Part model, mm, in its own coordinate system. Face numbers are marked on the shaded views. A direction names the side the tool comes from. Give positions to 0.01 mm unless a question says otherwise; leave off trailing zeros. Loops run counter-clockwise (first coordinate to the right, second up) from the corner with the lowest first, then second, coordinate; pieces in that order, holes last. Notation, with made-up numbers: M -7,22.5 L 50,22.5 A19 ccw 50,33.5 Z; hole C 35.25,3.25 d3. An arc over 180 degrees is marked long. Answer in a Markdown table with one row per item.
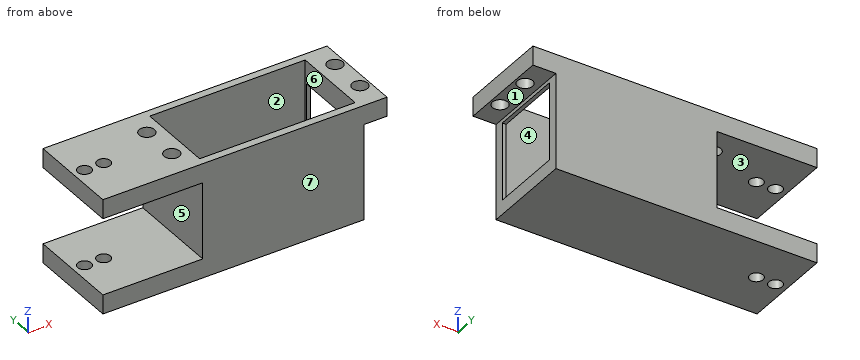
from build123d import *

# Parameters (mm, degrees)
SKETCH1_W                 = 56
SKETCH1_H                 = 24
BOSS_EXTRUDE1_DEPTH       = 30
SHELL1_T                  = -2
SHELL1_THICKNESS_2_FACE_W = 28
SHELL1_THICKNESS_2_FACE_H = 20
SHELL1_THICKNESS_2_DEPTH  = 6.5
SHELL1_THICKNESS_3_FACE_W = 28
SHELL1_THICKNESS_3_FACE_H = 20
SHELL1_THICKNESS_3_DEPTH  = 5
SKETCH12_W                = 20
SKETCH12_H                = 19
CUT_EXTRUDE1_DEPTH        = 10
FILLET1_R                 = 2
SKETCH13_W                = 2
SKETCH13_H                = 24
CUT_EXTRUDE2_DEPTH        = 43.755116653
SKETCH17_W                = 25
SKETCH17_H                = 24
CUT_EXTRUDE4_DEPTH        = 4
SKETCH19_R                = 2
CUT_EXTRUDE5_DEPTH        = 13
CUT_EXTRUDE7_DEPTH        = 2
SKETCH21_W                = 25
SKETCH21_H                = 24
CUT_EXTRUDE8_DEPTH        = 6
SKETCH26_W                = 5
SKETCH26_H                = 24
BOSS_EXTRUDE3_DEPTH       = 20
SKETCH27_W                = 5
SKETCH27_H                = 24
BOSS_EXTRUDE4_DEPTH       = 26
SKETCH28_R                = 1.75
CUT_EXTRUDE9_DEPTH        = 57.21387729


with BuildPart() as part:
    # Sketch1 → Boss-Extrude1 (new body)
    with BuildSketch(Plane.XY):
        Rectangle(SKETCH1_W, SKETCH1_H)
    extrude(amount=BOSS_EXTRUDE1_DEPTH)

    # Shell1
    shell1_openings = [part.faces().sort_by_distance(p)[0] for p in [
        (0, 0, 30),
    ]]
    offset(amount=SHELL1_T, openings=shell1_openings, kind=Kind.INTERSECTION)

    # Shell1 thickness 2 face (on inner face of the shell) → Shell1 thickness 2 (add)
    with BuildSketch(Plane(origin=(-26, 0, 16), x_dir=(0, 0, -1), z_dir=(-1, 0, 0))):
        Rectangle(SHELL1_THICKNESS_2_FACE_W, SHELL1_THICKNESS_2_FACE_H)
    extrude(amount=-SHELL1_THICKNESS_2_DEPTH)

    # Shell1 thickness 3 face (on inner face of the shell) → Shell1 thickness 3 (add)
    with BuildSketch(Plane(origin=(26, 0, 16), x_dir=(0, 0, 1), z_dir=(1, 0, 0))):
        Rectangle(SHELL1_THICKNESS_3_FACE_W, SHELL1_THICKNESS_3_FACE_H)
    extrude(amount=-SHELL1_THICKNESS_3_DEPTH)

    # Sketch12 → Cut-Extrude1 (cut)
    with BuildSketch(Plane(origin=(28, 0, 0), x_dir=(0, 0, -1), z_dir=(1, 0, 0))):
        with Locations((-14, 0)):
            Rectangle(SKETCH12_W, SKETCH12_H)
    extrude(amount=-CUT_EXTRUDE1_DEPTH, mode=Mode.SUBTRACT)

    # Fillet1
    fillet1_edges = [part.edges().sort_by_distance(p)[0] for p in [
        (21, 0, 4),
    ]]
    fillet(fillet1_edges, radius=FILLET1_R - 0.0001)  # a hair under: the kernel refuses the full size

    # Sketch13 → Cut-Extrude2 (cut, through all)
    with BuildSketch(Plane.XY.offset(30)):
        with Locations((-27, 0)):
            Rectangle(SKETCH13_W, SKETCH13_H)
    extrude(amount=-CUT_EXTRUDE2_DEPTH, mode=Mode.SUBTRACT)

    # Sketch17 → Cut-Extrude4 (cut)
    with BuildSketch(Plane(origin=(28, 0, 0), x_dir=(0, 0, -1), z_dir=(1, 0, 0))):
        with Locations((-12.5, 0)):
            Rectangle(SKETCH17_W, SKETCH17_H)
    extrude(amount=-CUT_EXTRUDE4_DEPTH, mode=Mode.SUBTRACT)

    # Sketch19 → Cut-Extrude5 (cut)
    with BuildSketch(Plane.XY.offset(30)):
        with Locations((-23.5, -5)):
            Circle(SKETCH19_R)
        with Locations((-23.5, 5)):
            Circle(SKETCH19_R)
        with Locations((25.5, 5)):
            Circle(SKETCH19_R)
        with Locations((25.5, -5)):
            Circle(SKETCH19_R)
    extrude(amount=-CUT_EXTRUDE5_DEPTH, mode=Mode.SUBTRACT)

    # Sketch20 → Cut-Extrude7 (cut)
    with BuildSketch(Plane(origin=(24, 0, 0), x_dir=(0, 0, -1), z_dir=(1, 0, 0))):
        Polygon((-25, 6.322875656), (-25, 12), (0, 12), (0, -12), (-25, -12), (-25, -6.322875656), align=None)
        Polygon((-24, -6.322875656), (-24, -9.5), (-4, -9.5), (-4, 9.5), (-24, 9.5), (-24, 6.322875656), align=None, mode=Mode.SUBTRACT)
    extrude(amount=-CUT_EXTRUDE7_DEPTH, mode=Mode.SUBTRACT)

    # Sketch21 → Cut-Extrude8 (cut)
    with BuildSketch(Plane.ZY.offset(26)):
        with Locations((12.5, 0)):
            Rectangle(SKETCH21_W, SKETCH21_H)
    extrude(amount=-CUT_EXTRUDE8_DEPTH, mode=Mode.SUBTRACT)

    # Sketch26 → Boss-Extrude3 (add)
    with BuildSketch(Plane.ZY.offset(26)):
        with Locations((27.5, 0)):
            Rectangle(SKETCH26_W, SKETCH26_H)
    extrude(amount=BOSS_EXTRUDE3_DEPTH)

    # Sketch27 → Boss-Extrude4 (add)
    with BuildSketch(Plane.ZY.offset(20)):
        with Locations((2.5, 0)):
            Rectangle(SKETCH27_W, SKETCH27_H)
    extrude(amount=BOSS_EXTRUDE4_DEPTH)

    # Sketch28 → Cut-Extrude9 (cut, through all)
    with BuildSketch(Plane.XY.offset(30)):
        with Locations((-43, 0)):
            Circle(SKETCH28_R)
        with Locations((-38, 0)):
            Circle(SKETCH28_R)
    extrude(amount=-CUT_EXTRUDE9_DEPTH, mode=Mode.SUBTRACT)


solid = part.part
(1) Saw through at B-B (x = -23.5). Write the cut outline in (y, z), plus the area to 3 significant figures.
Recorded:
| item | result |
|---|---|
| outline | M -12,0 L 12,0 L 12,5 L -12,5 Z; M -12,25 L -7,25 L -7,30 L -12,30 Z; M -3,25 L 3,25 L 3,30 L -3,30 Z; M 7,25 L 12,25 L 12,30 L 7,30 Z |
| area | 200 mm^2 |
(2) Which spindle directions (+Z, -Z, +X, -X, +Y, -Y) get a long thin tool onto all of the face, cutting with end or side? Do the marked faces 1, 2 and 3. Say none if no direction does.
Recorded:
| item | result |
|---|---|
| face 1 | -Z, +X, +Y, -Y |
| face 2 | +Z |
| face 3 | -X, +Y, -Y |
(3) Drill centre lines: line 1 along Y through (x, z) = (25.5, 27.4); line 2 along Y through (x, z) = (-38, 27.65); line 3 along Y through (x, z) = (-19, 15). Where is each one in solid material? Low to high.
Recorded:
| item | result |
|---|---|
| line 1 | y = -12 to -7, -3 to 3, 7 to 12 |
| line 2 | y = -12 to -1.75, 1.75 to 12 |
| line 3 | y = -12 to -10, 10 to 12 |
(4) Saw through at A-A (y = 0). Give the number of separate pieces and of enclosed holes in the cut face, plus the area to 3 significant figures.
Recorded:
| item | result |
|---|---|
| separate pieces | 6 |
| enclosed holes | 0 |
| area | 325 mm^2 |
(5) Pin check, flat tips, straight feed: pin 1 Ø10 at (y, z) = (2, 15.5) entering from +X; pin 2 Ø5 at (x, y) = (-11, 7) entering from +Z; pin 3 Ø5 at (x, y) = (25.5, -5) entering from -Z. Stop position of each tip, or through.
Recorded:
| item | result |
|---|---|
| pin 1 | stops at x = -19.5 |
| pin 2 | stops at z = 2 |
| pin 3 | stops at z = 25 |
(6) Saw through at C-C (z = 26.25). Write the cut outline in (x, y).
Recorded:
| item | result |
|---|---|
| outline | M -46,-12 L 28,-12 L 28,12 L -46,12 Z; hole C -43,0 d3.5; hole C -38,0 d3.5; hole C -23.5,-5 d4; hole C -23.5,5 d4; hole M -19.5,-10 L 21,-10 L 21,10 L -19.5,10 Z; hole C 25.5,-5 d4; hole C 25.5,5 d4 |
(7) Pull direction X, two halves, no side cores. Call the marked faces 4, 5, 6 and 7: +X half, -X half, draft (parallel to the pull), parting line (faces both ways), or undercut.
Recorded:
| item | result |
|---|---|
| face 4 | undercut |
| face 5 | -X half |
| face 6 | undercut |
| face 7 | draft |
